```python
from build123d import *

# Parameters (mm, degrees)
F0_W        = 80.6
F0_H        = 12
F1_DEPTH    = 2
F2_W        = 2
F2_H        = 9.2
F3_DEPTH    = 4.5
F4_W        = 9.2
F4_H        = 2.2
F5_DEPTH    = 0.8
F6_R        = 1.99999
F7_W        = 9.2
F7_H        = 2.2
F8_DEPTH    = 0.8
F9_T1_DEPTH = 14.0989794856
F9_T3_DEPTH = 14.2


# Not quite as in the source:
# - a fillet or chamfer that OpenCascade refuses, or shapes differently, is made with other operations: its cross-section is extruded or revolved along the edge and cut away or added
# - a fillet or chamfer is up to 0.001 mm smaller than in the source, because OpenCascade refuses the exact size


with BuildPart() as f1:
    # F0 (on Top) → F1 (new body)
    with BuildSketch(Plane.XY):
        with Locations((-40.3, 6)):
            Rectangle(F0_W, F0_H)
    extrude(amount=-F1_DEPTH)

    # F2 (on face) → F3 (join)
    with BuildSketch(Plane.XY):
        with Locations((-74.015, 7.4)):
            Rectangle(F2_W, F2_H)
        with Locations((-6.585, 7.4)):
            Rectangle(F2_W, F2_H)
    extrude(amount=F3_DEPTH)

    # F4 (on face) → F5 (join)
    with BuildSketch(Plane(origin=(-75.015, 0, 0), x_dir=(0, -1, 0), z_dir=(-1, 0, 0))):
        with Locations((-7.4, 3.4)):
            Rectangle(F4_W, F4_H)
    extrude(amount=F5_DEPTH)

    # F6 (radius 2 in the source; OpenCascade refuses exactly that, so slightly less here)
    f6_edges = [f1.edges().sort_by_distance(p)[0] for p in [
        (-80.6, 6, -2),
        (0, 6, -2),
        (-40.3, 0, -2),
    ]]
    fillet(f6_edges, radius=F6_R)

    # F7 (on face) → F8 (join)
    with BuildSketch(Plane.YZ.offset(-5.585)):
        with Locations((7.4, 3.4)):
            Rectangle(F7_W, F7_H)
    extrude(amount=F8_DEPTH)

    # F9: fillet of radius 1 on 4 edges, made by hand

    # F9_s2 → F9_t1 (cut)
    with BuildSketch(Plane.XZ.offset(-14.4494897428)):
        with BuildLine():
            ThreePointArc((-5.585, 2.3), (-5.0104033308, 2.6473403651), (-4.785, 3.2797958971))
            Line((-4.785, 3.2797958971), (-4.785, 2.3))
            Line((-4.785, 2.3), (-5.585, 2.3))
        make_face()
        with BuildLine():
            ThreePointArc((-75.815, 3.2797958971), (-75.5895966692, 2.6473403651), (-75.015, 2.3))
            Line((-75.015, 2.3), (-75.815, 2.3))
            Line((-75.815, 2.3), (-75.815, 3.2797958971))
        make_face()
    extrude(amount=F9_T1_DEPTH, mode=Mode.SUBTRACT)

    # F9_s4 → F9_t3 (cut)
    with BuildSketch(Plane.XZ.offset(-14.5)):
        with BuildLine():
            ThreePointArc((-4.785, 3.5), (-5.0778932188, 4.2071067812), (-5.785, 4.5))
            Line((-5.785, 4.5), (-4.785, 4.5))
            Line((-4.785, 4.5), (-4.785, 3.5))
        make_face()
        with BuildLine():
            ThreePointArc((-74.815, 4.5), (-75.5221067812, 4.2071067812), (-75.815, 3.5))
            Line((-75.815, 3.5), (-75.815, 4.5))
            Line((-75.815, 4.5), (-74.815, 4.5))
        make_face()
    extrude(amount=F9_T3_DEPTH, mode=Mode.SUBTRACT)


solid = f1.part
```
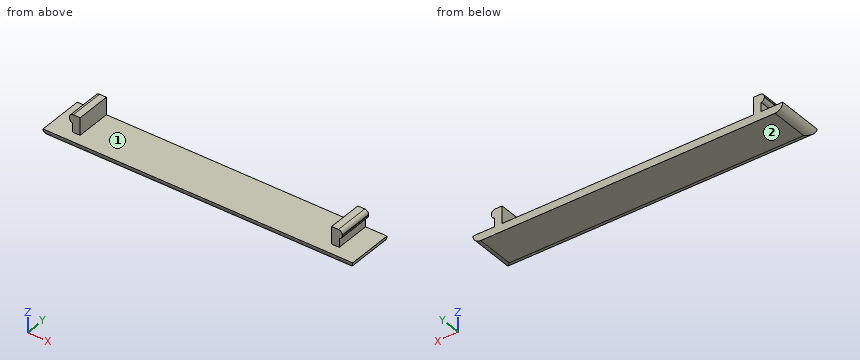
The model under review builds one solid part; all positions refer to its coordinate system, in mm. Face numbers are marked on the shaded views. Round coordinates to 2 decimals unless told otherwise and drop trailing zeros. Write each loop counter-clockwise with the first axis right and the second up, starting at its lowest first coordinate (ties: lowest second). Pieces come first, ordered by that corner, then holes.
(1) We need section A-A on z = 1. Give the boundary of the cut face in (x, y) (3 decimals).
(2) Wall thickness on L1, parallel to X at y = 6.25, z = 2 (3 decimals); L2, parallel to X at y = 11.5, z = 3.25 (3 decimals); L3, parallel to Z at x = -34.5, y = 7.75: over which ranges is each line inside the solid? List them lowest first.
(3) Mouldability with a two-part tool opening along X and no side actions: class the marked faces 1 and 2 as +X half, -X half, draft (parallel to the pull), parting line (faces both ways), or undercut.
(4) Insertion check: pin 1 (1.5 mm diameter, centred on x = -17.5, z = -0.5, fed in from -Y); pin 2 (0.8 mm diameter, centred on x = -74, z = 2, fed in from -Y); pin 3 (1.3 mm diameter, centred on y = 8, z = 2, fed in from -X); pin 4 (6 mm diameter, centred on x = -18, y = 8, fed in from +Z). Each pin has a flat end and moves straight along its axis. Give the tip position at first contact, or say it passes through.
Findings below:
1. outline: (-75.015, 2.8) - (-73.015, 2.8) - (-73.015, 12) - (-75.015, 12) - close; (-7.585, 2.8) - (-5.585, 2.8) - (-5.585, 12) - (-7.585, 12) - close
2. L1: x = -75.015 to -73.015, -7.585 to -5.585
2. L2: x = -75.815 to -73.015, -7.585 to -4.785
2. L3: z = -2 to 0
3. face 1: undercut
3. face 2: draft
4. pin 1: stops at y = 0
4. pin 2: stops at y = 2.8
4. pin 3: stops at x = -75.59
4. pin 4: stops at z = 0
